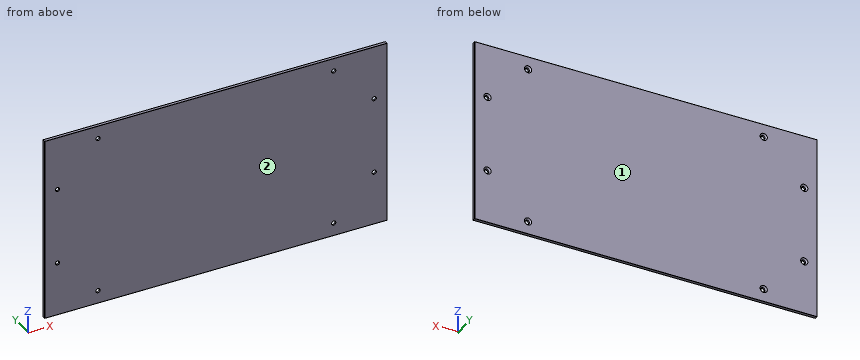
```python
from build123d import *

# Parameters (mm, degrees)
SKETCH1_W           = 642
SKETCH1_H           = 342
BOSS_EXTRUDE1_DEPTH = 6
SKETCH2_R           = 4
CUT_EXTRUDE1_DEPTH  = 7
CHAMFER1_SIZE       = 2.75
FILLET1_R           = 0.2


with BuildPart() as part:
    # Sketch1 → Boss-Extrude1 (new body)
    with BuildSketch(Plane(origin=(0, 0, 0), x_dir=(1, 0, 0), z_dir=(0, 1, 0))):
        Rectangle(SKETCH1_W, SKETCH1_H)
    extrude(amount=BOSS_EXTRUDE1_DEPTH)

    # Sketch2 → Cut-Extrude1 (cut, through all)
    with BuildSketch(Plane(origin=(0, 6, 0), x_dir=(1, 0, 0), z_dir=(0, 1, 0))):
        with Locations((-221, -147)):
            Circle(SKETCH2_R)
        with Locations((221, -147)):
            Circle(SKETCH2_R)
        with Locations((-297, -71)):
            Circle(SKETCH2_R)
        with Locations((297, -71)):
            Circle(SKETCH2_R)
        with Locations((297, 71)):
            Circle(SKETCH2_R)
        with Locations((221, 147)):
            Circle(SKETCH2_R)
        with Locations((-221, 147)):
            Circle(SKETCH2_R)
        with Locations((-297, 71)):
            Circle(SKETCH2_R)
    extrude(amount=-CUT_EXTRUDE1_DEPTH, mode=Mode.SUBTRACT)

    # Chamfer1
    chamfer1_edges = [part.edges().sort_by_distance(p)[0] for p in [
        (-225, 6, 147),
        (217, 6, 147),
        (-301, 6, 71),
        (293, 6, 71),
        (293, 6, -71),
        (217, 6, -147),
        (-225, 6, -147),
        (-301, 6, -71),
    ]]
    chamfer(chamfer1_edges, length=CHAMFER1_SIZE)

    # Fillet1
    fillet1_edges = [part.edges().sort_by_distance(p)[0] for p in [
        (-321, 6, 0),
        (0, 6, 171),
        (321, 6, 0),
        (0, 0, 171),
        (-321, 0, 0),
        (0, 0, -171),
        (321, 0, 0),
        (0, 6, -171),
        (321, 3, 171),
        (-321, 3, 171),
        (-321, 3, -171),
        (321, 3, -171),
    ]]
    fillet(fillet1_edges, radius=FILLET1_R)


solid = part.part
```
Here's how the part is built. I have some questions about the finished solid (model axes, mm). Face numbers are marked on the shaded views. Coordinates: 2 decimals unless noted, no trailing zeros. Answer as a JSON object with one key per item and string values. Group by question number.
(1) For pin 1 (13 mm diameter, centred on x = -297, z = -71, fed in from +Y); pin 2 (13 mm diameter, centred on x = 221, z = 147, fed in from -Y); pin 3 (10.5 mm diameter, centred on x = 221, z = -147, fed in from +Y), each with a flat end and sliding along its axis, tell me the tip position at first contact or that it passes through.
(2) I need wall thicknesses on probe 1 along X at (y, z) = (2.25, 71); probe 2 along Z at (x, y) = (-221, 0.8); probe 3 along Z at (x, y) = (297, 2.15). Which ranges of each line are inside material? Lowest first, please.
(3) If we mould it in two halves opening along Y, with no side actions, what happens to the marked faces 1 and 2? For each: released by +Y, released by -Y, zero draft, split by the parting line, or undercut.
Values found:
{
 "1": {"pin 1": "stops at y = 5.75", "pin 2": "stops at y = 0", "pin 3": "stops at y = 4.5"},
 "2": {"probe 1": "x = -321 to -301, -293 to 293, 301 to 321", "probe 2": "z = -171 to -151, -143 to 143, 151 to 171", "probe 3": "z = -171 to -75, -67 to 67, 75 to 171"},
 "3": {"face 1": "released by +Y", "face 2": "released by -Y"}
}
